Work out the finished part from the listing and answer in its coordinate system (mm). Coordinates: 2 decimals unless noted, no trailing zeros. Write each loop counter-clockwise with the first axis right and the second up, starting at its lowest first coordinate (ties: lowest second). Pieces come first, ordered by that corner, then holes. Notation, with made-up numbers: M 73.25,-2.5 L 119.25,-2.5 A24 ccw 119.25,28.5 Z; hole C 54.5,-33.5 d2. An arc over 180 degrees is marked long. Use CSV: the item, a comma, the result in double quotes.
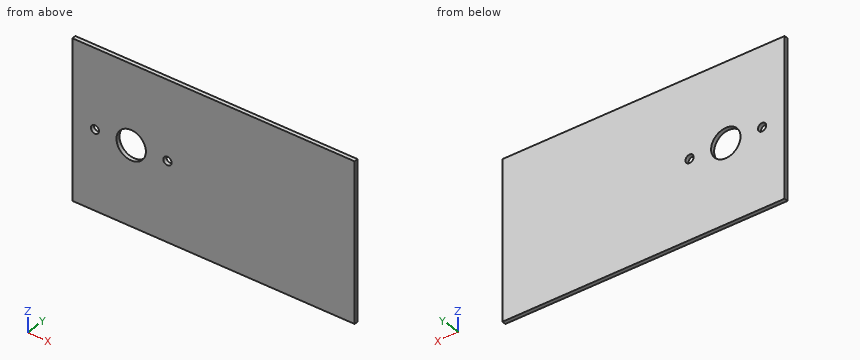
Autodesk Inventor part; units mm, degrees
ref_plane "YZ Plane" through (0, 0, 0) normal (1, 0, 0) x (0, 1, 0)
ref_plane "XZ Plane" through (0, 0, 0) normal (0, 1, 0) x (-1, 0, 0)
ref_plane "XY Plane" through (0, 0, 0) normal (0, 0, 1) x (1, 0, 0)
sketch "スケッチ1" plane through (0, 0, 0) normal (0, 1, 0) x (-1, 0, 0)
  line L0 (-70, 40) -> (70, 40)
  line L1 (70, 40) -> (70, -40)
  line L2 (70, -40) -> (-70, -40)
  line L3 (-70, -40) -> (-70, 40)
  line L4 (-70, 40) -> (70, -40) construction
  line L5 (70, 40) -> (-70, -40) construction
  point P0 (0, 0)
  dimension "d0" = 140
  dimension "d1" = 80
extrude "押し出し1" add sketch "スケッチ1" along normal blind 2
sketch "スケッチ2" plane through (0, 2, 0) normal (0, 1, 0) x (1, 0, 0)
  circle A0 centre (-40, 0) radius 7.5
  circle A1 centre (-58.5, 0) radius 2.1
  circle A2 centre (-21.5, 0) radius 2.1
  line L0 (70, 40) -> (70, -40)
  point P0 (0, 0)
  dimension "d4" = 15
  dimension "d6" = 4.2
  dimension "d7" = 4.2
  dimension "d8" = 37
  dimension "d9" = 18.5
  dimension "d12" = 110
extrude "押し出し2" cut sketch "スケッチ2" against normal blind 8
sketch "スケッチ3" plane through (70, 0, 40) normal (1, 0, 0) x (0, 0, -1)
  line L0 (0, 2) -> (80, 2)
  line L1 (0, 0) -> (80, 0)
  line L2 (80, 0) -> (80, 2)
  line L3 (80, 2) -> (0, 2)
  line L4 (0, 2) -> (0, 0)
  point P0 (40, 0)
extrude "押し出し3" add sketch "スケッチ3" along normal blind 4
properties part number "sholder_2" material "アルミニウム 6061"
Item 1: Given pin 1 (5.5 mm diameter, centred on x = -58.5, z = 0, fed in from -Y); pin 2 (4 mm diameter, centred on x = -21.5, z = 0, fed in from +Y), each flat-ended and moving along its own axis, determine where each tip first touches the part or whether it passes through.
Answer:
pin 1,"stops at y = 0"
pin 2,"passes through"
Item 2: The part is cut by section A-A (x = -40). Write down the section's boundary in (y, z).
Answer:
outline,"M 0,-40 L 2,-40 L 2,-7.5 L 0,-7.5 Z; M 0,7.5 L 2,7.5 L 2,40 L 0,40 Z"
Item 3: The part is cut by section C-C (y = 1.05). Write down the section's boundary in (x, z).
Answer:
outline,"M -70,-40 L 74,-40 L 74,40 L -70,40 Z; hole C -58.5,0 d4.2; hole C -40,0 d15; hole C -21.5,0 d4.2"
Item 4: The part is cut by section D-D (x = -21.5). Write down the section's boundary in (y, z), then the cut area to 3 significant figures.
Answer:
outline,"M 0,-40 L 2,-40 L 2,-2.1 L 0,-2.1 Z; M 0,2.1 L 2,2.1 L 2,40 L 0,40 Z"
area,"152 mm2"
Item 5: Consider probe 1 along X at (y, z) = (1.1, 0); probe 2 along Z at (x, y) = (-58.5, 1.5); probe 3 along Z at (x, y) = (-40.5, 1.4). Determine where each line is inside the solid, lowest interval first.
Answer:
probe 1,"x = -70 to -60.6, -56.4 to -47.5, -32.5 to -23.6, -19.4 to 74"
probe 2,"z = -40 to -2.1, 2.1 to 40"
probe 3,"z = -40 to -7.48, 7.48 to 40"
Item 6: The part is cut by section B-B (z = 0). Write down the section's boundary in (x, y), then the cut area to 3 significant figures.
Answer:
outline,"M -70,0 L -60.6,0 L -60.6,2 L -70,2 Z; M -56.4,0 L -47.5,0 L -47.5,2 L -56.4,2 Z; M -32.5,0 L -23.6,0 L -23.6,2 L -32.5,2 Z; M -19.4,0 L 74,0 L 74,2 L -19.4,2 Z"
area,"241 mm2"
